from build123d import *

# Parameters (mm, degrees)
SKETCH1_R                = 76.2
BOSS_EXTRUDE1_DEPTH      = 11.43
FILLET1_R                = 2.54
BOSS_EXTRUDE2_DEPTH      = 9.525
BOSS_EXTRUDE2_DEPTH_BACK = 20.955
SKETCH3_R                = 7.9375
FILLET2_R                = 1.27
CUT_EXTRUDE1_DEPTH       = 110.78156512
CUT_EXTRUDE1_DEPTH_BACK  = 110.78156512
SKETCH2_W                = 9.921875
SKETCH2_H                = 9.921875


with BuildPart() as part:
    # Sketch1 → Boss-Extrude1 (new body)
    with BuildSketch(Plane(origin=(0, 0, 0), x_dir=(1, 0, 0), z_dir=(0, 1, 0))):
        with Locations(Location((0, 0, 0), (0, 0, 270))):
            Circle(SKETCH1_R)
    extrude(amount=BOSS_EXTRUDE1_DEPTH)

    # Fillet1
    fillet1_edges = [part.edges().sort_by_distance(p)[0] for p in [
        (0, 0, -76.2),
        (0, 11.43, -76.2),
    ]]
    fillet(fillet1_edges, radius=FILLET1_R)

    # Sketch3 → Boss-Extrude2 (add, two sides: drawn at the far end of the back side and taken through both)
    with BuildSketch(Plane(origin=(0, 11.43, 0), x_dir=(1, 0, 0), z_dir=(0, 1, 0)).offset(-BOSS_EXTRUDE2_DEPTH_BACK)):
        with Locations(Location((0, 0, 0), (0, 0, 270))):
            Circle(SKETCH3_R)
    extrude(amount=BOSS_EXTRUDE2_DEPTH + BOSS_EXTRUDE2_DEPTH_BACK)

    # Fillet2
    fillet2_edges = [part.edges().sort_by_distance(p)[0] for p in [
        (0, 11.43, -7.9375),
        (0, 0, -7.9375),
    ]]
    fillet(fillet2_edges, radius=FILLET2_R)

    # Sketch2 → Cut-Extrude1 (cut, two sides: drawn at the far end of the back side and taken through both)
    with BuildSketch(Plane(origin=(0, 11.43, 0), x_dir=(1, 0, 0), z_dir=(0, 1, 0)).offset(-CUT_EXTRUDE1_DEPTH_BACK)):
        Rectangle(SKETCH2_W, SKETCH2_H)
    extrude(amount=CUT_EXTRUDE1_DEPTH + CUT_EXTRUDE1_DEPTH_BACK, mode=Mode.SUBTRACT)


solid = part.part
Could you check a few things on this model? Use its own coordinates, in mm. A direction names the side the tool comes from. Coordinates: 2 decimals unless noted, no trailing zeros. Order: outer loops, then holes, each group sorted by start corner. A loop starts at its lowest first (then second) coordinate and runs counter-clockwise, first axis right, second up. Notation, with made-up numbers: (48.25, 82.5) - (83.25, 82.5) arc R25 ccw to (83.25, 113.5) - close; hole circle Ø11 at (0, 84). An arc over 180 degrees is marked (long way). Answer in a Markdown table with one row per item. Add a question column.
(1) I need wall thicknesses on L1, parallel to Y at x = -46, z = -26; L2, parallel to Z at x = 2, y = 10.5; L3, parallel to Z at x = -6, y = 18. Which ranges of each line are inside material? Lowest first, please.
(2) If we section it at D-D, the plane y = -7.5: Please give me the cut outline in (x, z) (1 decimal), then the cut area to 3 significant figures.
(3) On a 3-axis mill with a long thin cutter (end or side, diameter ignored), from which of +Z, -Z, +X, -X, +Y, -Y can I reach the whole of each face in a straight line? I mean faces 1 (the face through (-4.961, 6, 0)), 2 (the face through (-7.75, -5.46, -1.72)), 3 (the face through (-5.2, -9.525, -0.1)). Say none if no direction works.
(4) If we mould it in two halves opening along Z, with no side actions, what happens to faces 4 (the face through (0, 6, -4.961)), 5 (the face through (-15, 0, -1)), 6 (the face through (4.961, 6, 0)), 7 (the face through (-7.75, 16.77, -1.72))? For each: released by +Z, released by -Z, zero draft, split by the parting line, or undercut.
(5) If we section it at B-B, the plane z = 0: Please give me the cut outline in (x, y) (1 decimal).
(6) If we section it at A-A, the plane x = 0: Please give me the cut outline in (y, z) (1 decimal).
(7) Will these pins go through, and if not, where does the flat tip stop? pin 1 (5 mm diameter, centred on y = 11, z = 1.5, fed in from +X); pin 2 (8 mm diameter, centred on y = 1.5, z = -1.5, fed in from -X); pin 3 (3 mm diameter, centred on x = 45.5, z = 33, fed in from -Y); pin 4 (8 mm diameter, centred on x = 37, y = -5, fed in from -Z).
(8) If we section it at C-C, the plane y = 7: Please give me the cut outline in (x, z), then the cut area to 3 significant figures.
Results are:
| question | item | result |
|---|---|---|
| 1 | L1 | y = 0 to 11.43 |
| 1 | L2 | z = -75.6 to -4.96, 4.96 to 75.6 |
| 1 | L3 | z = -5.2 to 5.2 |
| 2 | outline | circle Ø15.9 at (0, 0); hole (-5, -5) - (5, -5) - (5, 5) - (-5, 5) - close |
| 2 | area | 99.5 mm2 |
| 3 | face 1 | +Y, -Y |
| 3 | face 2 | -Y |
| 3 | face 3 | +Z, -Z, +X, -X, -Y |
| 4 | face 4 | undercut |
| 4 | face 5 | zero draft |
| 4 | face 6 | undercut |
| 4 | face 7 | split by the parting line |
| 5 | outline | (-76.2, 2.5) arc R2.5 ccw to (-73.7, 0) - (-9.2, 0) arc R1.3 cw to (-7.9, -1.3) - (-7.9, -9.5) - (-5, -9.5) - (-5, 21) - (-7.9, 21) - (-7.9, 12.7) arc R1.3 cw to (-9.2, 11.4) - (-73.7, 11.4) arc R2.5 ccw to (-76.2, 8.9) - close; (5, -9.5) - (7.9, -9.5) - (7.9, -1.3) arc R1.3 cw to (9.2, 0) - (73.7, 0) arc R2.5 ccw to (76.2, 2.5) - (76.2, 8.9) arc R2.5 ccw to (73.7, 11.4) - (9.2, 11.4) arc R1.3 cw to (7.9, 12.7) - (7.9, 21) - (5, 21) - close |
| 6 | outline | (-9.5, -7.9) - (-1.3, -7.9) arc R1.3 cw to (0, -9.2) - (0, -73.7) arc R2.5 ccw to (2.5, -76.2) - (8.9, -76.2) arc R2.5 ccw to (11.4, -73.7) - (11.4, -9.2) arc R1.3 cw to (12.7, -7.9) - (21, -7.9) - (21, -5) - (-9.5, -5) - close; (-9.5, 5) - (21, 5) - (21, 7.9) - (12.7, 7.9) arc R1.3 cw to (11.4, 9.2) - (11.4, 73.7) arc R2.5 ccw to (8.9, 76.2) - (2.5, 76.2) arc R2.5 ccw to (0, 73.7) - (0, 9.2) arc R1.3 cw to (-1.3, 7.9) - (-9.5, 7.9) - close |
| 7 | pin 1 | stops at x = 76.2 |
| 7 | pin 2 | stops at x = -76.2 |
| 7 | pin 3 | stops at y = 0 |
| 7 | pin 4 | passes through |
| 8 | outline | circle Ø152.4 at (0, 0); hole (-4.96, -4.96) - (4.96, -4.96) - (4.96, 4.96) - (-4.96, 4.96) - close |
| 8 | area | 18,100 mm2 |
